Work out the finished part from the listing and answer in its coordinate system (mm). Face numbers are marked on the shaded views. A direction names the side the tool comes from. Round coordinates to 2 decimals unless told otherwise and drop trailing zeros. Order: outer loops, then holes, each group sorted by start corner. A loop starts at its lowest first (then second) coordinate and runs counter-clockwise, first axis right, second up. Notation, with made-up numbers: (16, 33) -> (33, 33) arc R26 ccw to (33, 69) -> close; hole circle Ø6 at (-37.75, -10). An arc over 180 degrees is marked (long way). Use one line per item in the form item = value.
Autodesk Inventor part; units mm, degrees
ref_plane "YZ Plane" through (0, 0, 0) normal (1, 0, 0) x (0, 1, 0)
ref_plane "XZ Plane" through (0, 0, 0) normal (0, 1, 0) x (-1, 0, 0)
ref_plane "XY Plane" through (0, 0, 0) normal (0, 0, 1) x (1, 0, 0)
sketch "Sketch1" plane through (0, 0, 0) normal (0, 0, 1) x (1, 0, 0)
  line L0 (-12.5, 12.5) -> (12.5, 12.5)
  line L1 (12.5, 12.5) -> (12.5, -12.5)
  line L2 (12.5, -12.5) -> (-12.5, -12.5)
  line L3 (-12.5, -12.5) -> (-12.5, 12.5)
  point P0 (0, 0)
  dimension "d2" = 25
  dimension "d3" = 12.5
  dimension "d4" = 25
  dimension "d5" = 12.5
extrude "Extrusion1" add sketch "Sketch1" along normal blind 10
sketch "Sketch2" plane through (-12.5, 12.5, 0) normal (0, 1, 0) x (1, 0, 0)
  line L0 (25, -10) -> (0, -10)
  line L1 (25, 0) -> (0, 0)
  line L2 (0, 0) -> (0, -10)
  point P0 (12.5, 0)
  point P1 (4.5, -5)
  dimension "d8" = 10
  dimension "d9" = 5
  dimension "d18" = 8
hole "Hole1" at (-8, 12.5, 5) direction (0, -1, 0) diameter 4 depth 25
mirror "Mirror1" about plane through (0, 0, 0) normal (1, 0, 0) of "Hole1"
sketch "Sketch3" plane through (-12.5, -12.5, 0) normal (0, -1, 0) x (1, 0, 0)
  line L0 (0, 0) -> (25, 0)
  line L1 (0, 10) -> (25, 10)
  line L2 (0, 0) -> (0, 10)
  line L3 (25, 0) -> (25, 10)
  point P0 (12.5, 0)
  point P1 (12.5, 5)
  dimension "d19" = 10
  dimension "d20" = 25
  dimension "d21" = 12.5
  dimension "d22" = 5
hole "Hole2" at (0, -12.5, 5) direction (0, 1, 0) diameter 8 depth 20
chamfer "Chamfer1" distance 0.5 angle 45 1 edges at (0, -12.5, 9)
fillet "Fillet1" radius 2 4 edges at (-12.5, -12.5, 5) (-12.5, 12.5, 5) (12.5, 12.5, 5) (12.5, -12.5, 5)
properties part number "pendulum_mass" material "ABS Plastic"
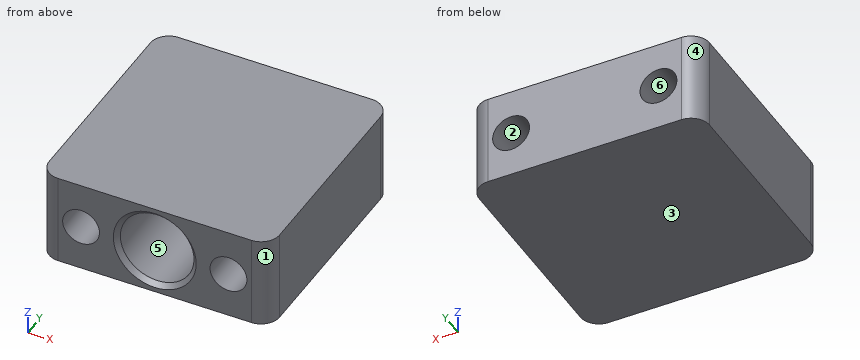
Item 1: Determine the mould class of the marked faces 1, 2, 3 and 4 for opening direction X: released by +X, released by -X, zero draft, split by the parting line, or undercut.
Findings:
face_1 = released by +X
face_2 = undercut
face_3 = zero draft
face_4 = released by -X
Item 2: The part is cut by section C-C, the plane y = -1.75. Give the vertices of the cut face in (x, z), and give its area (3 significant figures).
Findings:
outline = (-12.5, 0) -> (12.5, 0) -> (12.5, 10) -> (-12.5, 10) -> close; hole circle Ø4 at (-8, 5); hole circle Ø8 at (0, 5); hole circle Ø4 at (8, 5)
area = 175 mm^2
Item 3: Consider line 1 along X through (y, z) = (-7, 5); line 2 along Z through (x, y) = (0, -1); line 3 along X through (y, z) = (5.75, 4). Determine where each line is inside the solid, lowest interval first.
Findings:
line_1 = -12.5 to -10, -6 to -4, 4 to 6, 10 to 12.5
line_2 = 0 to 1, 9 to 10
line_3 = -12.5 to -9.73, -6.27 to -3.87, 3.87 to 6.27, 9.73 to 12.5
Item 4: For the marked faces 5 and 6, determine the directions among +Z, -Z, +X, -X, +Y, -Y from which every point of the face is accessible in a straight line to the end or side of a thin tool.
Findings:
face_5 = -Y
face_6 = +Y, -Y
Item 5: The part is cut by section B-B, the plane x = 8. Give the vertices of the cut face in (y, z), and give its area (3 significant figures).
Findings:
outline = (-12.5, 0) -> (12.5, 0) -> (12.5, 3) -> (-12.5, 3) -> close; (-12.5, 7) -> (12.5, 7) -> (12.5, 10) -> (-12.5, 10) -> close
area = 150 mm^2
Item 6: The part is cut by section A-A, the plane z = 5. Give the vertices of the cut face in (x, y).
Findings:
outline = (-12.5, -10.5) arc R2 ccw to (-10.5, -12.5) -> (-10, -12.5) -> (-10, 12.5) -> (-10.5, 12.5) arc R2 ccw to (-12.5, 10.5) -> close; (-6, -12.5) -> (-4.5, -12.5) -> (-4, -12) -> (-4, 7.5) -> (4, 7.5) -> (4, -12) -> (4.5, -12.5) -> (6, -12.5) -> (6, 12.5) -> (-6, 12.5) -> close; (10, -12.5) -> (10.5, -12.5) arc R2 ccw to (12.5, -10.5) -> (12.5, 10.5) arc R2 ccw to (10.5, 12.5) -> (10, 12.5) -> close
Item 7: The part is cut by section D-D, the plane x = 0. Give the vertices of the cut face in (y, z).
Findings:
outline = (-12.5, 0) -> (12.5, 0) -> (12.5, 10) -> (-12.5, 10) -> (-12.5, 9.5) -> (-12, 9) -> (7.5, 9) -> (7.5, 1) -> (-12, 1) -> (-12.5, 0.5) -> close
